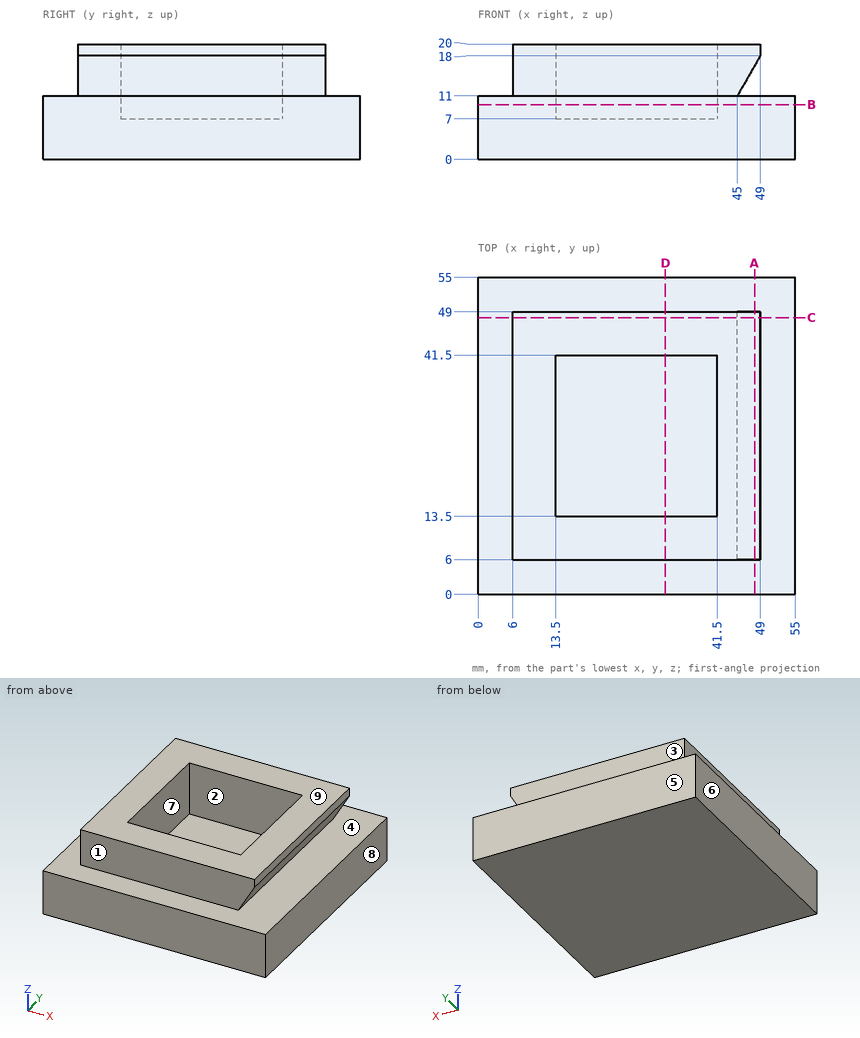
Here's the drawing with two shaded views (mm, measured from the low corner). I have some questions. A direction names the side the tool comes from. Round coordinates to 2 decimals unless told otherwise and drop trailing zeros. Loops run counter-clockwise (first coordinate to the right, second up) from the corner with the lowest first, then second, coordinate; pieces in that order, holes last.
Item 1: Suppose I cut it at D-D, the plane x = 32.5. Write out the boundary of the cut face in (y, z), then the cut area to 3 significant figures.
Item 2: Which directions (+Z, -Z, +X, -X, +Y, -Y) give clear straight access to the entire face, cutting with the end or side of a thin tool? Please do the marked faces 1, 2, 3, 4 and 5.
Item 3: Please list where these lines run through material, in increasing order: L1, parallel to Y at x = 31, z = 11.5; L2, parallel to Y at x = 20.5, z = 9.75; L3, parallel to Z at x = 52, y = 12.5.
Item 4: Suppose I cut it at A-A, the plane x = 48. Write out the boundary of the cut face in (y, z).
Item 5: If we mould it in two halves opening along X, with no side actions, what happens to the marked faces 6, 7, 8 and 9? For each: +X half, -X half, draft (parallel to the pull), parting line (faces both ways), or undercut.
Item 6: Suppose I cut it at B-B, the plane z = 9.5. Write out the boundary of the cut face in (x, y).
Item 7: Suppose I cut it at C-C, the plane y = 48. Write out the boundary of the cut face in (x, z), then the cut area to 3 significant figures.
Item 8: Will these pins go through, and if not, where does the flat tip stop? pin 1 Ø5 at (x, y) = (32.5, 22) entering from +Z; pin 2 Ø7 at (x, z) = (34.5, 17.5) entering from +Y; pin 3 Ø5 at (y, z) = (26, 17) entering from -X.
Reported:
1. outline: (0, 0) - (55, 0) - (55, 11) - (49, 11) - (49, 20) - (41.5, 20) - (41.5, 7) - (13.5, 7) - (13.5, 20) - (6, 20) - (6, 11) - (0, 11) - close
1. area: 628 mm2
2. face 1: +Z, +X, -X, -Y
2. face 2: +Z
2. face 3: +Z, +X, -X, +Y
2. face 4: none
2. face 5: +Z, -Z, +X, -X, +Y
3. L1: y = 6 to 13.5, 41.5 to 49
3. L2: y = 0 to 13.5, 41.5 to 55
3. L3: z = 0 to 11
4. outline: (0, 0) - (55, 0) - (55, 11) - (0, 11) - close; (6, 16.25) - (49, 16.25) - (49, 20) - (6, 20) - close
5. face 6: -X half
5. face 7: undercut
5. face 8: +X half
5. face 9: draft
6. outline: (0, 0) - (55, 0) - (55, 55) - (0, 55) - close; hole (13.5, 13.5) - (41.5, 13.5) - (41.5, 41.5) - (13.5, 41.5) - close
7. outline: (0, 0) - (55, 0) - (55, 11) - (45, 11) - (49, 18) - (49, 20) - (6, 20) - (6, 11) - (0, 11) - close
7. area: 978 mm2
8. pin 1: stops at z = 7
8. pin 2: stops at y = 49
8. pin 3: stops at x = 6
